```python
from build123d import *

# Parameters (mm, degrees)
F0_W      = 63.5
F0_H      = 44.45
F1_DEPTH  = 38.1
F2_W      = 25.4
F2_H      = 38.1
F3_DEPTH  = 38.1
F4_W      = 19.05
F4_H      = 38.1
F5_DEPTH  = 38.1
F6_R      = 3.175
F7_DEPTH  = 25.4
F9_DEPTH  = 25.4
F11_DEPTH = 25.4
F12_R     = 6.35
F13_DEPTH = 25.4


with BuildPart() as f1:
    # F0 (on Front) → F1 (new body)
    with BuildSketch(Plane.XZ):
        with Locations((31.75, 22.225)):
            Rectangle(F0_W, F0_H)
    extrude(amount=F1_DEPTH)

    # F2 (on face) → F3 (cut)
    with BuildSketch(Plane.XZ.offset(38.1)):
        with Locations((50.8, 25.4)):
            Rectangle(F2_W, F2_H)
    extrude(amount=-F3_DEPTH, mode=Mode.SUBTRACT)

    # F4 (on face) → F5 (cut)
    with BuildSketch(Plane.YZ.offset(38.1)):
        with Locations((-28.575, 25.4)):
            Rectangle(F4_W, F4_H)
    extrude(amount=-F5_DEPTH, mode=Mode.SUBTRACT)

    # F6 (on face) → F7 (cut)
    with BuildSketch(Plane.XY.offset(6.35)):
        with Locations((53.975, -9.525)):
            Circle(F6_R)
        with Locations((53.975, -28.575)):
            Circle(F6_R)
        with Locations((9.525, -28.575)):
            Circle(F6_R)
    extrude(amount=-F7_DEPTH, mode=Mode.SUBTRACT)

    # F8 (on face) → F9 (cut)
    with BuildSketch(Plane.XY.offset(6.35)):
        with BuildLine():
            ThreePointArc((7.6932702214, -38.1), (2.5225699869, -35.7128573059), (0, -30.6068577154))
            Line((0, -30.6068577154), (0, -38.1))
            Line((0, -38.1), (7.6932702214, -38.1))
        make_face()
        with BuildLine():
            ThreePointArc((63.5, -31.6278859973), (59.9629765941, -36.172141291), (54.536730051, -38.1))
            Line((54.536730051, -38.1), (63.5, -38.1))
            Line((63.5, -38.1), (63.5, -31.6278859973))
        make_face()
    extrude(amount=-F9_DEPTH, mode=Mode.SUBTRACT)

    # F10 (on face) → F11 (cut)
    with BuildSketch(Plane.XZ.offset(19.05)):
        with BuildLine():
            ThreePointArc((0, 34.2015661299), (12.7, 41.9675576974), (25.4, 34.2015661299))
            Line((25.4, 34.2015661299), (25.4, 14.0428527725))
            ThreePointArc((25.4, 14.0428527725), (30.6758841641, 8.4231867937), (38.1, 6.35))
            Line((38.1, 6.35), (38.1, 44.45))
            Line((38.1, 44.45), (0, 44.45))
            Line((0, 44.45), (0, 34.2015661299))
        make_face()
    extrude(amount=-F11_DEPTH, mode=Mode.SUBTRACT)

    # F12 (on face) → F13 (cut)
    with BuildSketch(Plane.XZ.offset(19.05)):
        with Locations((12.7, 27.7001828811)):
            Circle(F12_R)
    extrude(amount=-F13_DEPTH, mode=Mode.SUBTRACT)


solid = f1.part
```
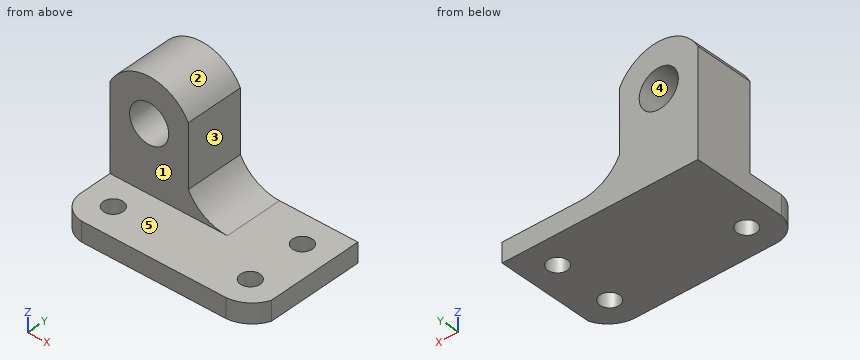
For this review, take the finished solid that the model builds, in its own axes (mm). Face numbers are marked on the shaded views. A direction names the side the tool comes from. Give positions to 0.01 mm unless a question says otherwise; leave off trailing zeros. Write each loop counter-clockwise with the first axis right and the second up, starting at its lowest first coordinate (ties: lowest second). Pieces come first, ordered by that corner, then holes. Notation, with made-up numbers: M 16.25,-34 L 29.25,-34 A3 ccw 29.25,-29 Z; hole C 10.5,44 d6. An arc over 180 degrees is marked long. Answer as a JSON object with one key per item and string values. Group by question number.
Item 1: Tool access review of the marked faces 1 and 2: name each direction out of +Z, -Z, +X, -X, +Y, -Y from which nothing blocks a thin tool from reaching the whole face with its end or side.
Item 2: Consider section B-B on x = 55.5. Write out the cut boundary in (y, z), plus the area to 3 significant figures.
Item 3: Consider section C-C on z = 16. Write out the cut boundary in (x, y).
Item 4: For pin 1 Ø7.5 at (x, y) = (53.975, -9.525) entering from -Z; pin 2 Ø1 at (x, z) = (19, 7) entering from -Y; pin 3 Ø5.5 at (y, z) = (-13.5, 21.5) entering from +X; pin 4 Ø8.5 at (x, y) = (53.975, -28.575) entering from +Z, all flat-tipped, find the tip position at first contact; note any pin that passes through.
Item 5: Consider section A-A on x = 17.5. Write out the cut boundary in (y, z), plus the area to 3 significant figures.
Item 6: Draft analysis for pull direction X (two halves, no side actions). For the marked faces 3, 4 and 5, state which applies: +X half, -X half, draft (parallel to the pull), parting line (faces both ways), or undercut.
Item 7: For probe 1 along Z at (x, y) = (12.7, -11.75); probe 2 along Z at (x, y) = (55, -17); probe 3 along X at (y, z) = (-6, 16), list the stretches that pass through material, from the lowest coordinate up. Write a range as [from, to].
Item 8: Consider section D-D on y = -22.5. Write out the cut boundary in (x, z), plus the area to 3 significant figures.
Check result:
{
 "1": {"face 1": "+Z, +X, -X, -Y", "face 2": "+Z, +Y, -Y"},
 "2": {"outline": "M -38,0 L -31.36,0 L -31.36,6.35 L -38,6.35 Z; M -25.79,0 L -12.31,0 L -12.31,6.35 L -25.79,6.35 Z; M -6.74,0 L 0,0 L 0,6.35 L -6.74,6.35 Z", "area": "171 mm^2"},
 "3": {"outline": "M 0,-19.05 L 25.4,-19.05 L 25.4,0 L 0,0 Z"},
 "4": {"pin 1": "stops at z = 0", "pin 2": "stops at y = -19.05", "pin 3": "stops at x = 25.4", "pin 4": "stops at z = 6.35"},
 "5": {"outline": "M -38.1,0 L 0,0 L 0,23.54 L -19.05,23.54 L -19.05,6.35 L -38.1,6.35 Z; M -19.05,31.86 L 0,31.86 L 0,41.14 L -19.05,41.14 Z", "area": "746 mm^2"},
 "6": {"face 3": "+X half", "face 4": "undercut", "face 5": "draft"},
 "7": {"probe 1": "z = [0, 21.35], [34.05, 41.97]", "probe 2": "z = [0, 6.35]", "probe 3": "x = [0, 25.4]"},
 "8": {"outline": "M 0,0 L 63.5,0 L 63.5,6.35 L 0,6.35 Z", "area": "403 mm^2"}
}
